Part model, mm, in its own coordinate system. A direction names the side the tool comes from. Round coordinates to 2 decimals unless told otherwise and drop trailing zeros. Loops run counter-clockwise (first coordinate to the right, second up) from the corner with the lowest first, then second, coordinate; pieces in that order, holes last.
(1) Probe probe 1 along X at (y, z) = (-70, 20); probe 2 along Z at (x, y) = (-13, -19.5); probe 3 along X at (y, z) = (-66, 25.75). List the from-to ranges inside material, lowest first.
(2) Cut at A-A on y = -73.5. List the corners of the cut face in (x, z).
(3) Tool access for faces 1 (the face through (-49.687, -50, 24)), 2 (the face through (-14, -50, 28.288)): list every direction of +Z, -Z, +X, -X, +Y, -Y with a clear straight run to the whole face (end or side of a thin tool).
(4) Cut at B-B on z = 15.5. List the corners of the cut face in (x, y).
(5) Flat gauge pin, fed straight in: pin 1 (12 mm diameter, centred on x = -16, y = -67, fed in from -Z). Where does the tip first touch, or does it go through?
(6) Cut at C-C on x = -36.5. List the corners of the cut face in (y, z).
(7) Cut at D-D on x = -26. List the corners of the cut face in (y, z).
from build123d import *

# Parameters (mm, degrees)
F1_DEPTH = 101.6


with BuildPart() as f1:
    # F0 (on Front) → F1 (new body)
    with BuildSketch(Plane.XZ):
        Polygon((23.185539, 34.638372), (-49.687061, 34.638372), (-49.687061, 28.288372), (-32.948462, 28.288372), (-23.702861, 28.288372), (-2.798661, 28.288372), (6.446939, 28.288372), (23.185539, 28.288372), align=None)
        with BuildLine():
            Line((-32.948462, 28.288372), (-49.687061, 28.288372))
            Line((-49.687061, 28.288372), (-49.687061, 20.261972))
            Line((-49.687061, 20.261972), (-40.974861, 20.261972))
            ThreePointArc((-40.974861, 20.261972), (-38.623983, 25.937493), (-32.948462, 28.288372))
        make_face()
        with BuildLine():
            Line((-40.974861, 20.261972), (-49.687061, 20.261972))
            Line((-49.687061, 20.261972), (-49.687061, 12.235572))
            Line((-49.687061, 12.235572), (-32.948461, 12.235572))
            ThreePointArc((-32.948461, 12.235572), (-38.623983, 14.58645), (-40.974861, 20.261972))
        make_face()
        with BuildLine():
            Line((23.185539, 20.261972), (23.185539, 28.288372))
            Line((23.185539, 28.288372), (6.446939, 28.288372))
            ThreePointArc((6.446939, 28.288372), (12.12246, 25.937493), (14.473339, 20.261972))
            Line((14.473339, 20.261972), (23.185539, 20.261972))
        make_face()
        with BuildLine():
            Line((23.185539, 12.235572), (23.185539, 20.261972))
            Line((23.185539, 20.261972), (14.473339, 20.261972))
            ThreePointArc((14.473339, 20.261972), (12.12246, 14.58645), (6.446939, 12.235572))
            Line((6.446939, 12.235572), (23.185539, 12.235572))
        make_face()
    extrude(amount=F1_DEPTH)


solid = f1.part
Final values:
1. probe 1: x = -49.69 to -40.97, 14.47 to 23.19
1. probe 2: z = 28.29 to 34.64
1. probe 3: x = -49.69 to -38.81, 12.3 to 23.19
2. outline: (-49.69, 12.24) - (-32.95, 12.24) arc R8.03 cw to (-40.97, 20.26) arc R8.03 cw to (-32.95, 28.29) - (6.45, 28.29) arc R8.03 cw to (14.47, 20.26) arc R8.03 cw to (6.45, 12.24) - (23.19, 12.24) - (23.19, 34.64) - (-49.69, 34.64) - close
3. face 1: +Z, -Z, -X, +Y, -Y
3. face 2: -Z, +Y, -Y
4. outline: (-49.69, -101.6) - (-39.41, -101.6) - (-39.41, 0) - (-49.69, 0) - close; (12.91, -101.6) - (23.19, -101.6) - (23.19, 0) - (12.91, 0) - close
5. pin 1: stops at z = 28.29
6. outline: (-101.6, 12.24) - (0, 12.24) - (0, 13.06) - (-101.6, 13.06) - close; (-101.6, 27.46) - (0, 27.46) - (0, 34.64) - (-101.6, 34.64) - close
7. outline: (-101.6, 28.29) - (0, 28.29) - (0, 34.64) - (-101.6, 34.64) - close
